The listing builds one solid part. Answer for the finished solid, in the listing's coordinates (mm). Face numbers are marked on the shaded views. Coordinates: 2 decimals unless noted, no trailing zeros. Order: outer loops, then holes, each group sorted by start corner. A loop starts at its lowest first (then second) coordinate and runs counter-clockwise, first axis right, second up. Notation, with made-up numbers: (62, 2) -> (99, 2) arc R18 cw to (99, 29) -> close; hole circle Ø10 at (45.5, 59.25). An arc over 180 degrees is marked (long way). Return JSON: item names as keys, results as strings.
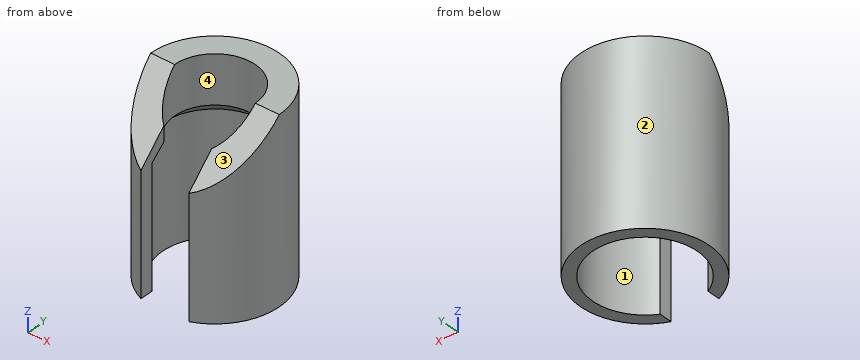
from build123d import *

# Parameters (mm, degrees)
F1_DEPTH      = 10
F3_DEPTH      = 5
F4_SIZE       = 0.99999
F6_DEPTH      = 25
F6_DEPTH_BACK = 25


# Not quite as in the source:
# - a fillet or chamfer is up to 0.001 mm smaller than in the source, because OpenCascade refuses the exact size


with BuildPart() as f1:
    # F0 (on Top) → F1 (new body)
    with BuildSketch(Plane.XY):
        with BuildLine():
            Line((2, -3.8910956041), (2, -4.9890505109))
            ThreePointArc((2, -4.9890505109), (0, 5.375), (-2, -4.9890505109))
            Line((-2, -4.9890505109), (-2, -3.8910956041))
            ThreePointArc((-2, -3.8910956041), (0, 4.375), (2, -3.8910956041))
        make_face()
    extrude(amount=F1_DEPTH)

    # F2 (on face) → F3 (join)
    with BuildSketch(Plane.XY.offset(10)):
        with BuildLine():
            Line((2, -2.7185703964), (2, -4.9890505109))
            ThreePointArc((2, -4.9890505109), (0, 5.375), (-2, -4.9890505109))
            Line((-2, -4.9890505109), (-2, -2.7185703964))
            ThreePointArc((-2, -2.7185703964), (0, 3.375), (2, -2.7185703964))
        make_face()
    extrude(amount=F3_DEPTH)

    # F4 (size 1 in the source; OpenCascade refuses exactly that, so slightly less here)
    f4_edges = [f1.edges().sort_by_distance(p)[0] for p in [
        (0, 3.375, 10),
    ]]
    chamfer(f4_edges, length=F4_SIZE)

    # F5 (on Right) → F6 (cut, two sides)
    with BuildSketch(Plane.YZ) as f6_sk:
        Polygon((0, 15), (-4.9890505109, 15), (-4.9890505109, 10), align=None)
    extrude(amount=-F6_DEPTH, mode=Mode.SUBTRACT)
    extrude(f6_sk.sketch, amount=F6_DEPTH_BACK, mode=Mode.SUBTRACT)


solid = f1.part
1. Determine the mould class of the marked faces 1, 2, 3 and 4 for opening direction X: pulls with the +X half, pulls with the -X half, needs draft (parallel to the pull), parting line crosses it, or undercut.
Answer block:
{"face 1": "undercut", "face 2": "parting line crosses it", "face 3": "needs draft", "face 4": "undercut"}
2. The part is cut by section C-C on z = 13.5. Give the vertices of the cut face in (x, y) (3 decimals), and give its area (3 significant figures).
Answer block:
{"outline": "(-5.162, -1.497) -> (-3.025, -1.497) arc R3.375 cw (long way) to (3.025, -1.497) -> (5.162, -1.497) arc R5.375 ccw (long way) to start", "area": "33.6 mm2"}
3. The part is cut by section A-A on y = -4.5. Give the vertices of the cut face in (x, z).
Answer block:
{"outline": "(-2.94, 0) -> (-2, 0) -> (-2, 10.49) -> (-2.94, 10.49) -> close; (2, 0) -> (2.94, 0) -> (2.94, 10.49) -> (2, 10.49) -> close"}
4. Each of these flat-tipped pins is pushed along its axis until it touches: pin 1 Ø0.7 at (y, z) = (-3.5, 4) entering from +X; pin 2 Ø1.5 at (y, z) = (3.5, 9.5) entering from +X; pin 3 Ø1 at (y, z) = (1, 11) entering from -X. Where does it stop, or does it pass through?
Answer block:
{"pin 1": "stops at x = 4.36", "pin 2": "stops at x = 4.62", "pin 3": "stops at x = -5.35"}
5. The part is cut by section B-B on z = 1.25. Give the vertices of the cut face in (x, y) (3 decimals).
Answer block:
{"outline": "(-2, -4.989) -> (-2, -3.891) arc R4.375 cw (long way) to (2, -3.891) -> (2, -4.989) arc R5.375 ccw (long way) to start"}
6. Consider line 1 (X direction, y = 0, z = 12.55) (3 decimals); line 2 (Y direction, x = 0, z = 12.6) (3 decimals); line 3 (X direction, y = 0, z = 4.5) (3 decimals). Determine where each line is inside the solid, lowest interval first. Write a range as from..to.
Answer block:
{"line 1": "x = -5.375..-3.375, 3.375..5.375", "line 2": "y = 3.375..5.375", "line 3": "x = -5.375..-4.375, 4.375..5.375"}
